Geometry check sheet. Reference: the model listing, model coordinates, mm. Give positions to 0.01 mm unless a question says otherwise; leave off trailing zeros. Write each loop counter-clockwise with the first axis right and the second up, starting at its lowest first coordinate (ties: lowest second). Pieces come first, ordered by that corner, then holes. Notation, with made-up numbers: M -9.75,74 L 44.25,74 A7 cw 44.25,87 Z; hole C 86.25,21 d11. An arc over 180 degrees is marked long. Write each question's results on one line, items separated by ' | '.
```python
from build123d import *

# Parameters (mm, degrees)
F0_W     = 69
F0_H     = 15
F1_DEPTH = 5
F3_D     = 10
F5_D     = 4


with BuildPart() as f1:
    # F0 (on Top) → F1 (new body)
    with BuildSketch(Plane.XY):
        Rectangle(F0_W, F0_H)
    extrude(amount=F1_DEPTH)

    # F3 (through all)
    with Locations(Plane.XY.offset(5)):
        with Locations((-24.5, 0)):
            Hole(F3_D / 2)

    # F5 (through all)
    with Locations(Plane.XY.offset(5)):
        with Locations((12, 0), (27, 0)):
            Hole(F5_D / 2)


solid = f1.part
```
Q1. Section check B-B (x = -24.5). Enter the section's corners in (y, z).
Answer key:
outline: M -7.5,0 L -5,0 L -5,5 L -7.5,5 Z; M 5,0 L 7.5,0 L 7.5,5 L 5,5 Z
Q2. Section check A-A (y = 0). Enter the section's corners in (x, z), then the cut area to 3 significant figures.
Answer key:
outline: M -34.5,0 L -29.5,0 L -29.5,5 L -34.5,5 Z; M -19.5,0 L 10,0 L 10,5 L -19.5,5 Z; M 14,0 L 25,0 L 25,5 L 14,5 Z; M 29,0 L 34.5,0 L 34.5,5 L 29,5 Z | area: 255 mm2
Q3. Release check for a two-part mould opening along Y. For faces 1 (the face through (0, 7.5, 2)), 2 (the face through (25.092, 0.601, 2.465)), 3 (the face through (0, 0, 5)) record: released by +Y, released by -Y, zero draft, split by the parting line, or undercut.
Answer key:
face 1: released by +Y | face 2: undercut | face 3: zero draft
Q4. Material ranges on probe 1 along Y at (x, z) = (27, 1.85); probe 2 along X at (y, z) = (0.25, 0.8); probe 3 along X at (y, z) = (-0.5, 4.35), recorded low to high. Write a range as [from, to].
Answer key:
probe 1: y = [-7.5, -2], [2, 7.5] | probe 2: x = [-34.5, -29.49], [-19.51, 10.02], [13.98, 25.02], [28.98, 34.5] | probe 3: x = [-34.5, -29.47], [-19.53, 10.06], [13.94, 25.06], [28.94, 34.5]
Q5. Depth check by flat-ended pin: P1, Ø5, axis at x = -0.5, y = 5, coming from the -Z side. Enter the tip coordinate at first touch or a pass-through.
Answer key:
P1: stops at z = 0
Q6. Section check D-D (y = -2.75). Enter the section's corners in (x, z).
Answer key:
outline: M -34.5,0 L -28.68,0 L -28.68,5 L -34.5,5 Z; M -20.32,0 L 34.5,0 L 34.5,5 L -20.32,5 Z
Q7. Section check C-C (z = 1.85). Enter the section's corners in (x, y).
Answer key:
outline: M -34.5,-7.5 L 34.5,-7.5 L 34.5,7.5 L -34.5,7.5 Z; hole C -24.5,0 d10; hole C 12,0 d4; hole C 27,0 d4
